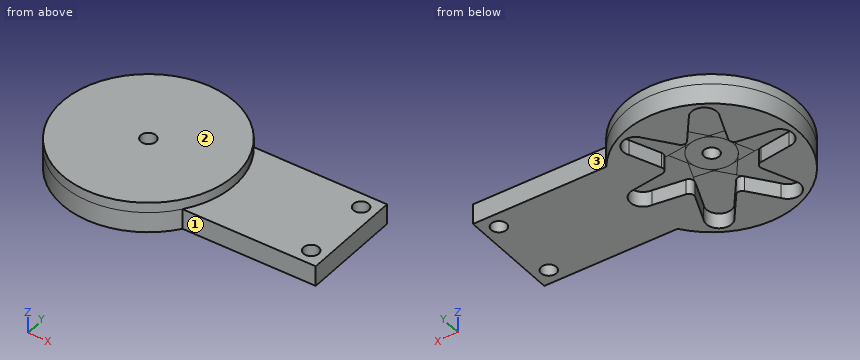
```python
from build123d import *

# Parameters (mm, degrees)
SKETCH1_W                       = 40
SKETCH1_H                       = 20
BOSS_EXTRUDE1_DEPTH             = 2
BOSS_EXTRUDE2_REACH             = 24.716
SKETCH6_R                       = 17
BOSS_EXTRUDE2_DIRECTION_2_DEPTH = 2
SKETCH7_R                       = 2.5
CUT_EXTRUDE3_DEPTH              = 3
CIRPATTERN1_COUNT               = 6
FILLET3_R                       = 1
CUT_EXTRUDE4_REACH              = 43.158
SKETCH8_R                       = 1.5
CUT_EXTRUDE5_REACH              = 42.915
SKETCH9_R                       = 1.5


with BuildPart() as part:
    # Sketch1 → Boss-Extrude1 (new, symmetric)
    with BuildSketch(Plane.XY):
        Rectangle(SKETCH1_W, SKETCH1_H)
    extrude(amount=BOSS_EXTRUDE1_DEPTH, both=True)

    # Boss-Extrude2: up to this face of the body (flat: up to its plane)
    boss_extrude2_end = Plane(part.part.faces().sort_by_distance((0, 0, -2))[0])
    # Sketch6 → Boss-Extrude2 (add, up to the picked face)
    with BuildSketch(Plane.XY.offset(2), mode=Mode.PRIVATE) as boss_extrude2_sk1:
        with Locations(Location((-20, 0, 0), (0, 0, 36.031879072))):
            Circle(SKETCH6_R)
    boss_extrude2_tool1 = split(extrude(boss_extrude2_sk1.sketch, amount=-BOSS_EXTRUDE2_REACH, mode=Mode.PRIVATE), bisect_by=boss_extrude2_end, keep=Keep.BOTH, mode=Mode.PRIVATE)
    add(boss_extrude2_tool1.solids().sort_by(Axis((-20, 0, 2), (0, 0, -1)))[0])

    # Sketch6 → Boss-Extrude2 direction 2 (add)
    with BuildSketch(Plane.XY.offset(2)):
        with Locations(Location((-20, 0, 0), (0, 0, 36.031879072))):
            Circle(SKETCH6_R)
    extrude(amount=BOSS_EXTRUDE2_DIRECTION_2_DEPTH)

    # Sketch7 → Cut-Extrude3 (cut)
    with BuildSketch(Plane(origin=(0, 0, -2), x_dir=(-1, 0, 0), z_dir=(0, 0, -1))):
        with BuildLine():
            Line((21.148365434, 4.169758006), (20, 4.325))
            ThreePointArc((20, 4.325), (15.675, 0), (20, -4.325))
            Line((20, -4.325), (21.148365434, -4.169758006))
            ThreePointArc((21.148365434, -4.169758006), (23.440371019, -2.620967808), (24.325, 0))
            ThreePointArc((24.325, 0), (23.440371019, 2.620967808), (21.148365434, 4.169758006))
        make_face()
        with BuildLine():
            Line((33.5, 2.5), (21.148365434, 4.169758006))
            ThreePointArc((21.148365434, 4.169758006), (23.440371019, 2.620967808), (24.325, 0))
            ThreePointArc((24.325, 0), (23.440371019, -2.620967808), (21.148365434, -4.169758006))
            Line((21.148365434, -4.169758006), (33.5, -2.5))
            ThreePointArc((33.5, -2.5), (31, 0), (33.5, 2.5))
        make_face()
        with Locations((33.5, 0)):
            Circle(SKETCH7_R)
    cut_extrude3 = extrude(amount=-CUT_EXTRUDE3_DEPTH, mode=Mode.SUBTRACT)

    # CirPattern1: Cut-Extrude3 ×6 about axis
    cirpattern1_axis = Axis((-20, 0, 0), (0, 0, 1))
    for i in range(1, CIRPATTERN1_COUNT):
        add(cut_extrude3.rotate(cirpattern1_axis, i * 360 / CIRPATTERN1_COUNT), mode=Mode.SUBTRACT)

    # Fillet3
    fillet3_edges = [part.edges().sort_by_distance(p)[0] for p in [
        (-26.069873399, 3.504443041, -0.5),
        (-20, 7.008886081, -0.5),
        (-13.930126601, 3.504443041, -0.5),
        (-13.930126601, -3.504443041, -0.5),
        (-20, -7.008886081, -0.5),
        (-26.069873399, -3.504443041, -0.5),
    ]]
    fillet(fillet3_edges, radius=FILLET3_R)

    # Sketch8 → Cut-Extrude4 (cut, up to next)
    with BuildSketch(Plane.XY.offset(4), mode=Mode.PRIVATE) as cut_extrude4_sk1:
        with Locations((-20, 0)):
            Circle(SKETCH8_R)
    cut_extrude4_tool1 = extrude(cut_extrude4_sk1.sketch, amount=-CUT_EXTRUDE4_REACH, mode=Mode.PRIVATE) & part.part
    add(cut_extrude4_tool1.solids().sort_by_distance((-20, 0, 4))[0], mode=Mode.SUBTRACT)

    # Sketch9 → Cut-Extrude5 (cut, up to next)
    with BuildSketch(Plane.XY.offset(2), mode=Mode.PRIVATE) as cut_extrude5_sk1:
        with Locations((17, 7)):
            Circle(SKETCH9_R)
    cut_extrude5_tool1 = extrude(cut_extrude5_sk1.sketch, amount=-CUT_EXTRUDE5_REACH, mode=Mode.PRIVATE) & part.part
    # Sketch9 → Cut-Extrude5 (cut, up to next)
    with BuildSketch(Plane.XY.offset(2), mode=Mode.PRIVATE) as cut_extrude5_sk2:
        with Locations((17, -7)):
            Circle(SKETCH9_R)
    cut_extrude5_tool2 = extrude(cut_extrude5_sk2.sketch, amount=-CUT_EXTRUDE5_REACH, mode=Mode.PRIVATE) & part.part
    add(cut_extrude5_tool1.solids().sort_by_distance((17, 7, 2))[0], mode=Mode.SUBTRACT)
    add(cut_extrude5_tool2.solids().sort_by_distance((17, -7, 2))[0], mode=Mode.SUBTRACT)


solid = part.part
```
Work out the finished part from the listing and answer in its coordinate system (mm). Face numbers are marked on the shaded views. A direction names the side the tool comes from. Give positions to 0.01 mm unless a question says otherwise; leave off trailing zeros. Loops run counter-clockwise (first coordinate to the right, second up) from the corner with the lowest first, then second, coordinate; pieces in that order, holes last. Notation, with made-up numbers: M -4.5,77.5 L -0.5,77.5 A25 cw -0.5,115.5 Z; hole C 72,-2.5 d1. An arc over 180 degrees is marked long. One line per item, written item: value. Start each with the question number.
1. Find the intervals of material crossed by probe 1 along Y at (x, z) = (17, 0.6); probe 2 along Y at (x, z) = (-20, 3.3); probe 3 along X at (y, z) = (-10.5, -1.4), in increasing order.
2. Find section B-B (z = -1.25). State how many separate pieces and enclosed holes the cut face has, and give its area (3 significant figures).
3. Which of the six approach directions +Z, -Z, +X, -X, +Y, -Y give full straight-line access (tool end or side, diameter ignored) to the marked faces 1, 2 and 3?
4. Each of these flat-tipped pins is pushed along its axis until it touches: P1, Ø2.5, axis at x = -33, y = -0.5, coming from the -Z side; P2, Ø1.8, axis at x = -20, y = 0, coming from the -Z side; P3, Ø2, axis at x = 10.5, z = -0.5, coming from the -Y side; P4, Ø2, axis at y = 12.5, z = 0.5, coming from the +X side. Where does it stop, or does it pass through?
5. Find section C-C (x = -1.5). Give the vertices of the cut face in (y, z), and give its area (3 significant figures).
6. Find section A-A (x = 17). Give the vertices of the cut face in (y, z).
7. Find section D-D (x = -10). Give the vertices of the cut face in (y, z).
Reported:
1. probe 1: y = -10 to -8.5, -5.5 to 5.5, 8.5 to 10
1. probe 2: y = -17 to -1.5, 1.5 to 17
1. probe 3: x = -33.37 to -28.95, -22.7 to -17.3, -11.05 to -6.63
2. separate pieces: 1
2. enclosed holes: 3
2. area: 918 mm²
3. face 1: +Z, -Z, +X, -Y
3. face 2: +Z, +X, -X, +Y, -Y
3. face 3: +Z, -Z, +X, +Y
4. P1: stops at z = 1
4. P2: passes through
4. P3: stops at y = -10
4. P4: stops at x = -7.48
5. outline: M -10,-2 L 10,-2 L 10,2 L -10,2 Z
5. area: 80.0 mm²
6. outline: M -10,-2 L -8.5,-2 L -8.5,2 L -10,2 Z; M -5.5,-2 L 5.5,-2 L 5.5,2 L -5.5,2 Z; M 8.5,-2 L 10,-2 L 10,2 L 8.5,2 Z
7. outline: M -13.75,-2 L -2.97,-2 L -2.97,1 L 2.97,1 L 2.97,-2 L 13.75,-2 L 13.75,4 L -13.75,4 Z
